from build123d import *

# Parameters (mm, degrees)
SKETCH_R      = 4
EXTRUDE_DEPTH = 40
FILLET_R      = 2
FILLET001_R   = 2


with BuildPart() as part:
    # Sketch → Extrude (new body)
    with BuildSketch(Plane.XZ):
        with BuildLine():
            Line((0, 0), (40, 0))
            Line((40, 0), (40, 10))
            Line((40, 10), (30, 10))
            Line((30, 10), (30, 15))
            ThreePointArc((30, 15), (20, 25), (10, 15))
            Line((10, 10), (10, 15))
            Line((0, 10), (10, 10))
            Line((0, 10), (0, 0))
        make_face()
        with Locations((20, 15)):
            Circle(SKETCH_R, mode=Mode.SUBTRACT)
    extrude(amount=EXTRUDE_DEPTH)

    # Fillet
    fillet_edges = [part.edges().sort_by_distance(p)[0] for p in [
        (40, -20, 10),
        (30, -20, 10),
        (10, -20, 10),
        (0, -20, 10),
    ]]
    fillet(fillet_edges, radius=FILLET_R)

    # Fillet001
    fillet001_edges = [part.edges().sort_by_distance(p)[0] for p in [
        (20, 0, 25),
        (16, 0, 15),
        (20, -40, 25),
        (16, -40, 15),
    ]]
    fillet(fillet001_edges, radius=FILLET001_R)


solid = part.part
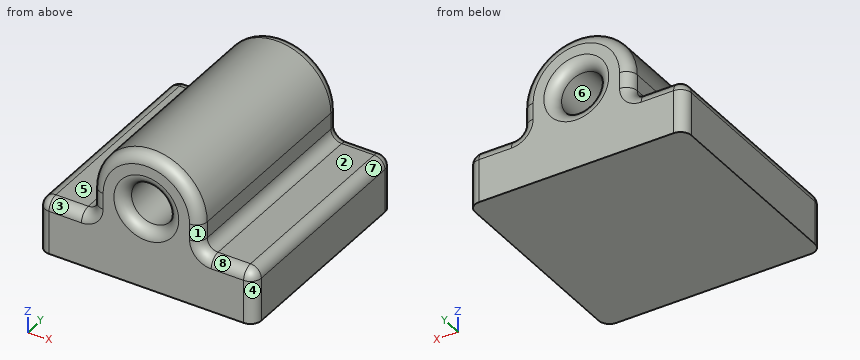
For this review, take the finished solid that the model builds, in its own axes (mm). Face numbers are marked on the shaded views. A direction names the side the tool comes from. Coordinates: 2 decimals unless noted, no trailing zeros. Order: outer loops, then holes, each group sorted by start corner. A loop starts at its lowest first (then second) coordinate and runs counter-clockwise, first axis right, second up. Notation, with made-up numbers: (51, 69) - (87, 69) arc R26 ccw to (87, 101) - close; hole circle Ø5 at (62, 9). An arc over 180 degrees is marked (long way). Answer as CSV lines item,"result". Start each with the question number.
1) Add section A-A (x = 20). State the section outline as (y, z) points.
2) To check wall thickness, follow line 1 along Z through (x, y) = (20, -12); line 2 along X through (y, z) = (-21.5, 14.5); line 3 along Z through (x, y) = (18.5, -28). State the ranges of each line that lie inside material, in increasing order. Write a range as [from, to].
3) Draft analysis for pull direction X (two halves, no side actions). For the marked faces 6, 7 and 8, state which applies: +X half, -X half, draft (parallel to the pull), parting line (faces both ways), or undercut.
4) Insertion check: P1, Ø10, axis at x = 11, y = -32.5, coming from the +Z side; P2, Ø5, axis at x = 34.5, y = -21, coming from the +Z side; P3, Ø6, axis at x = 34, y = -5, coming from the +Z side; P4, Ø1.5, axis at x = 12, z = 11, coming from the +Y side. Each pin has a flat end and moves straight along its axis. Give the tip position at first contact, or say it passes through.
5) Add section B-B (y = -32). State the section outline as (x, z) points.
6) Add section C-C (x = 34.5). State the section outline as (y, z) points.
7) Machinability: for the marked faces 1, 2, 3, 4 and 5, which of the approach directions +Z, -Z, +X, -X, +Y, -Y give a long, thin tool a straight path to every point of the face, cutting with its end or side? Answer none if there is none.
Result:
1,outline,"(-40, 0) - (0, 0) - (0, 9) arc R2 ccw to (-2, 11) - (-38, 11) arc R2 ccw to (-40, 9) - close; (-40, 21) arc R2 ccw to (-38, 19) - (-2, 19) arc R2 ccw to (0, 21) - (0, 23) arc R2 ccw to (-2, 25) - (-38, 25) arc R2 ccw to (-40, 23) - close"
2,line 1,"[0, 11], [19, 25]"
2,line 2,"[10, 16.03], [23.97, 30]"
2,line 3,"[0, 11.29], [18.71, 24.89]"
3,face 6,"undercut"
3,face 7,"+X half"
3,face 8,"draft"
4,P1,"z = 24.17"
4,P2,"z = 10"
4,P3,"z = 10.27"
4,P4,"y = 0"
5,outline,"(0, 0) - (40, 0) - (40, 8) arc R2 ccw to (38, 10) - (32, 10) arc R2 cw to (30, 12) - (30, 15) arc R10 ccw to (10, 15) - (10, 12) arc R2 cw to (8, 10) - (2, 10) arc R2 ccw to (0, 8) - close; hole circle Ø8 at (20, 15)"
6,outline,"(-40, 0) - (0, 0) - (0, 8) arc R2 ccw to (-2, 10) - (-38, 10) arc R2 ccw to (-40, 8) - close"
7,face 1,"+Z, +X, -Y"
7,face 2,"+Z, +X, +Y, -Y"
7,face 3,"+Z, -X, -Y"
7,face 4,"+Z, -Z, +X, -Y"
7,face 5,"+Z, -X, +Y, -Y"
